Could you check a few things on this model? Use its own coordinates, in mm. A direction names the side the tool comes from. Give positions to 0.01 mm unless a question says otherwise; leave off trailing zeros. Loops run counter-clockwise (first coordinate to the right, second up) from the corner with the lowest first, then second, coordinate; pieces in that order, holes last.
1. Imagine slicing it at D-D (x = -3.25). List the corners of the cut face in (y, z) for me, plus the area to 3 significant figures.
2. Imagine slicing it at A-A (y = 1.5). List the corners of the cut face in (x, z) for me, plus the area to 3 significant figures.
3. Thinking about a two-plate mould opening in X: for faces 1 (the flat face through (0, 0, 0)), 2 (the flat face through (-1.5, -7, 0)), 3 (the flat face through (2, -4, 0)), 4 (the flat face through (1.5, -7, 0)), which applies, +X half, -X half, draft (parallel to the pull), parting line (faces both ways), or undercut?
4. Imagine slicing it at B-B (z = 0). List the corners of the cut face in (x, y) for me, plus the area to 3 significant figures.
5. For faces 5 (the flat face through (-2, -2, -2)), 6 (the flat face through (0, -10, 0)), 7 (the flat face through (-2, -4, 0)), which set-ups out of +Z, -Z, +X, -X, +Y, -Y let a thin tool reach every point of the face, with its end or its side?
6. I need wall thicknesses on line 1 along X through (y, z) = (-7.5, 1.5); line 2 along Y through (x, z) = (2, 1); line 3 along Y through (x, z) = (0, 0). Which ranges of each line are inside material? Lowest first, please.
7. Imagine slicing it at C-C (y = -1). List the corners of the cut face in (x, z) for me, plus the area to 3 significant figures.
8. For P1, Ø1.5, axis at x = 2, z = 3.5, coming from the -Y side; P2, Ø4, axis at y = -7.5, z = -0.5, coming from the +X side; P3, Ø0.5, axis at x = -2, z = 0.5, coming from the -Y side; P4, Ø1.5, axis at x = -3, y = -6, coming from the -Z side, each with a flat end and sliding along its axis, tell me the tip position at first contact or that it passes through.
```python
from build123d import *

# Parameters (mm, degrees)
SKETCH1_R           = 3.95
BOSS_EXTRUDE1_DEPTH = 4
SKETCH2_R           = 4.4
BOSS_EXTRUDE2_DEPTH = 2
SKETCH4_R           = 2.4
BOSS_EXTRUDE3_DEPTH = 2
BOSS_EXTRUDE4_DEPTH = 6
SKETCH6_R           = 4.4
SKETCH6_R_2         = 3.95
BOSS_EXTRUDE5_DEPTH = 4
CUT_EXTRUDE1_DEPTH  = 4


with BuildPart() as part:
    # Sketch1 → Boss-Extrude1 (new body)
    with BuildSketch(Plane(origin=(0, 0, 0), x_dir=(1, 0, 0), z_dir=(0, 1, 0))):
        with Locations(Location((0, 0, 0), (0, 0, 270))):
            Circle(SKETCH1_R)
        with BuildLine():
            ThreePointArc((-0.166646614, 2.345141313), (-0.092401566, 2.286261662), (0, 2.2652595))
            ThreePointArc((0, 2.2652595), (0.092401566, 2.286261662), (0.166646614, 2.345141313))
            ThreePointArc((0.166646614, 2.345141313), (0.365153552, 2.422635524), (0.531999564, 2.290073216))
            ThreePointArc((0.531999564, 2.290073216), (0.585591031, 2.211925311), (0.667696959, 2.164620376))
            ThreePointArc((0.667696959, 2.164620376), (0.762183879, 2.157453631), (0.850485509, 2.191833312))
            ThreePointArc((0.850485509, 2.191833312), (1.063015161, 2.207373726), (1.183375246, 2.031522064))
            ThreePointArc((1.183375246, 2.031522064), (1.211551295, 1.941049689), (1.276066113, 1.871645232))
            ThreePointArc((1.276066113, 1.871645232), (1.364242809, 1.836946378), (1.458755034, 1.843771303))
            ThreePointArc((1.458755034, 1.843771303), (1.666423208, 1.795977086), (1.729602845, 1.592461261))
            ThreePointArc((1.729602845, 1.592461261), (1.72985991, 1.497703284), (1.771051193, 1.412366197))
            ThreePointArc((1.771051193, 1.412366197), (1.845082779, 1.353218377), (1.937407773, 1.331882123))
            ThreePointArc((1.937407773, 1.331882123), (2.121762239, 1.225), (2.12214764, 1.011903287))
            ThreePointArc((2.12214764, 1.011903287), (2.094462881, 0.92127937), (2.108670602, 0.827592226))
            ThreePointArc((2.108670602, 0.827592226), (2.161979047, 0.749250985), (2.243913329, 0.701649371))
            ThreePointArc((2.243913329, 0.701649371), (2.388573385, 0.545176288), (2.326130305, 0.341433266))
            ThreePointArc((2.326130305, 0.341433266), (2.272963633, 0.262995741), (2.258925375, 0.169283054))
            ThreePointArc((2.258925375, 0.169283054), (2.286773988, 0.078709355), (2.351037339, 0.009071994))
            ThreePointArc((2.351037339, 0.009071994), (2.443149303, -0.183088729), (2.323426084, -0.3593746))
            ThreePointArc((2.323426084, -0.3593746), (2.249501592, -0.418656214), (2.208464714, -0.504067659))
            ThreePointArc((2.208464714, -0.504067659), (2.208379026, -0.598825947), (2.249261363, -0.68431147))
            ThreePointArc((2.249261363, -0.68431147), (2.280640684, -0.89508551), (2.114275259, -1.028250455))
            ThreePointArc((2.114275259, -1.028250455), (2.026161462, -1.063108727), (1.961772273, -1.13262975))
            ThreePointArc((1.961772273, -1.13262975), (1.933759896, -1.223152935), (1.947628645, -1.316890857))
            ThreePointArc((1.947628645, -1.316890857), (1.915487132, -1.527550015), (1.717261799, -1.605761745))
            ThreePointArc((1.717261799, -1.605761745), (1.622787995, -1.613099364), (1.540767756, -1.660552716))
            ThreePointArc((1.540767756, -1.660552716), (1.487317713, -1.738797417), (1.472940575, -1.832458712))
            ThreePointArc((1.472940575, -1.832458712), (1.380134142, -2.024284997), (1.167662092, -2.040594058))
            ThreePointArc((1.167662092, -2.040594058), (1.075222693, -2.019759044), (0.982859262, -2.040928287))
            ThreePointArc((0.982859262, -2.040928287), (0.908720824, -2.099942118), (0.86737527, -2.185204569))
            ThreePointArc((0.86737527, -2.185204569), (0.722150177, -2.341153374), (0.514310485, -2.294110633))
            ThreePointArc((0.514310485, -2.294110633), (0.432119136, -2.246954269), (0.337619409, -2.239958423))
            ThreePointArc((0.337619409, -2.239958423), (0.249380102, -2.274497747), (0.184739867, -2.343785411))
            ThreePointArc((0.184739867, -2.343785411), (0, -2.45), (-0.184739867, -2.343785411))
            ThreePointArc((-0.184739867, -2.343785411), (-0.249380102, -2.274497747), (-0.337619409, -2.239958423))
            ThreePointArc((-0.337619409, -2.239958423), (-0.432119136, -2.246954269), (-0.514310485, -2.294110633))
            ThreePointArc((-0.514310485, -2.294110633), (-0.722150177, -2.341153374), (-0.86737527, -2.185204569))
            ThreePointArc((-0.86737527, -2.185204569), (-0.908720824, -2.099942118), (-0.982859262, -2.040928287))
            ThreePointArc((-0.982859262, -2.040928287), (-1.075222693, -2.019759044), (-1.167662092, -2.040594058))
            ThreePointArc((-1.167662092, -2.040594058), (-1.380134142, -2.024284997), (-1.472940575, -1.832458712))
            ThreePointArc((-1.472940575, -1.832458712), (-1.487317713, -1.738797417), (-1.540767756, -1.660552716))
            ThreePointArc((-1.540767756, -1.660552716), (-1.622787995, -1.613099364), (-1.717261799, -1.605761745))
            ThreePointArc((-1.717261799, -1.605761745), (-1.915487132, -1.527550015), (-1.947628645, -1.316890857))
            ThreePointArc((-1.947628645, -1.316890857), (-1.933759896, -1.223152935), (-1.961772273, -1.13262975))
            ThreePointArc((-1.961772273, -1.13262975), (-2.026161462, -1.063108727), (-2.114275259, -1.028250455))
            ThreePointArc((-2.114275259, -1.028250455), (-2.280640684, -0.89508551), (-2.249261363, -0.68431147))
            ThreePointArc((-2.249261363, -0.68431147), (-2.208379026, -0.598825947), (-2.208464714, -0.504067659))
            ThreePointArc((-2.208464714, -0.504067659), (-2.249501592, -0.418656214), (-2.323426084, -0.3593746))
            ThreePointArc((-2.323426084, -0.3593746), (-2.443149303, -0.183088729), (-2.351037339, 0.009071994))
            ThreePointArc((-2.351037339, 0.009071994), (-2.286773988, 0.078709355), (-2.258925375, 0.169283054))
            ThreePointArc((-2.258925375, 0.169283054), (-2.272963633, 0.262995741), (-2.326130305, 0.341433266))
            ThreePointArc((-2.326130305, 0.341433266), (-2.388573385, 0.545176288), (-2.243913329, 0.701649371))
            ThreePointArc((-2.243913329, 0.701649371), (-2.161979047, 0.749250985), (-2.108670602, 0.827592226))
            ThreePointArc((-2.108670602, 0.827592226), (-2.094462881, 0.92127937), (-2.12214764, 1.011903287))
            ThreePointArc((-2.12214764, 1.011903287), (-2.121762239, 1.225), (-1.937407773, 1.331882123))
            ThreePointArc((-1.937407773, 1.331882123), (-1.845082779, 1.353218377), (-1.771051193, 1.412366197))
            ThreePointArc((-1.771051193, 1.412366197), (-1.72985991, 1.497703284), (-1.729602845, 1.592461261))
            ThreePointArc((-1.729602845, 1.592461261), (-1.666423208, 1.795977086), (-1.458755034, 1.843771303))
            ThreePointArc((-1.458755034, 1.843771303), (-1.364242809, 1.836946378), (-1.276066113, 1.871645232))
            ThreePointArc((-1.276066113, 1.871645232), (-1.211551295, 1.941049689), (-1.183375246, 2.031522064))
            ThreePointArc((-1.183375246, 2.031522064), (-1.063015161, 2.207373726), (-0.850485509, 2.191833312))
            ThreePointArc((-0.850485509, 2.191833312), (-0.762183879, 2.157453631), (-0.667696959, 2.164620376))
            ThreePointArc((-0.667696959, 2.164620376), (-0.585591031, 2.211925311), (-0.531999564, 2.290073216))
            ThreePointArc((-0.531999564, 2.290073216), (-0.365153552, 2.422635524), (-0.166646614, 2.345141313))
        make_face(mode=Mode.SUBTRACT)
    extrude(amount=BOSS_EXTRUDE1_DEPTH)

    # Sketch2 → Boss-Extrude2 (add)
    with BuildSketch(Plane.XZ):
        with Locations(Location((0, 0, 0), (0, 0, 270))):
            Circle(SKETCH2_R)
    extrude(amount=BOSS_EXTRUDE2_DEPTH)

    # Sketch4 → Boss-Extrude3 (add)
    with BuildSketch(Plane.XZ.offset(2)):
        with Locations(Location((0, 0, 0), (0, 0, 270))):
            Circle(SKETCH4_R)
    extrude(amount=BOSS_EXTRUDE3_DEPTH)

    # Sketch5 → Boss-Extrude4 (add)
    with BuildSketch(Plane.XZ.offset(4)):
        with BuildLine():
            ThreePointArc((1.5, 1.8734994), (0, 2.4), (-1.5, 1.8734994))
            Line((-1.5, 1.8734994), (-1.5, -1.8734994))
            ThreePointArc((-1.5, -1.8734994), (0, -2.4), (1.5, -1.8734994))
            Line((1.5, -1.8734994), (1.5, 1.8734994))
        make_face()
    extrude(amount=BOSS_EXTRUDE4_DEPTH)

    # Sketch6 → Boss-Extrude5 (add)
    with BuildSketch(Plane(origin=(0, 0, 0), x_dir=(1, 0, 0), z_dir=(0, 1, 0))):
        with Locations(Location((0, 0, 0), (0, 0, 270))):
            Circle(SKETCH6_R)
        Circle(SKETCH6_R_2, mode=Mode.SUBTRACT)
    extrude(amount=BOSS_EXTRUDE5_DEPTH)

    # Sketch8 → Cut-Extrude1 (cut)
    with BuildSketch(Plane(origin=(0, 4, 0), x_dir=(1, 0, 0), z_dir=(0, 1, 0))):
        with BuildLine():
            ThreePointArc((0.746832801, 2.421172474), (0.402414119, 2.669843231), (0, 2.533739407))
            ThreePointArc((0, 2.533739407), (-0.402414119, 2.669843231), (-0.746832801, 2.421172474))
            ThreePointArc((-0.746832801, 2.421172474), (-1.171486096, 2.432615943), (-1.42730623, 2.093473742))
            ThreePointArc((-1.42730623, 2.093473742), (-1.836466392, 1.979240054), (-1.980957237, 1.579760681))
            ThreePointArc((-1.980957237, 1.579760681), (-2.33826859, 1.35), (-2.3585915, 0.92567895))
            ThreePointArc((-2.3585915, 0.92567895), (-2.632305363, 0.600806522), (-2.526654558, 0.189346583))
            ThreePointArc((-2.526654558, 0.189346583), (-2.692450252, -0.201771253), (-2.47021327, -0.563810059))
            ThreePointArc((-2.47021327, -0.563810059), (-2.513359121, -0.986420766), (-2.194282693, -1.266869704))
            ThreePointArc((-2.194282693, -1.266869704), (-2.110945003, -1.683422465), (-1.723380469, -1.857362415))
            ThreePointArc((-1.723380469, -1.857362415), (-1.520964157, -2.230844691), (-1.099348328, -2.282820325))
            ThreePointArc((-1.099348328, -2.282820325), (-0.795838971, -2.580046576), (-0.377634263, -2.505439631))
            ThreePointArc((-0.377634263, -2.505439631), (0, -2.7), (0.377634263, -2.505439631))
            ThreePointArc((0.377634263, -2.505439631), (0.795838971, -2.580046576), (1.099348328, -2.282820325))
            ThreePointArc((1.099348328, -2.282820325), (1.520964157, -2.230844691), (1.723380469, -1.857362415))
            ThreePointArc((1.723380469, -1.857362415), (2.110945003, -1.683422465), (2.194282693, -1.266869704))
            ThreePointArc((2.194282693, -1.266869704), (2.513359121, -0.986420766), (2.47021327, -0.563810059))
            ThreePointArc((2.47021327, -0.563810059), (2.692450252, -0.201771253), (2.526654558, 0.189346583))
            ThreePointArc((2.526654558, 0.189346583), (2.632305363, 0.600806522), (2.3585915, 0.92567895))
            ThreePointArc((2.3585915, 0.92567895), (2.33826859, 1.35), (1.980957237, 1.579760681))
            ThreePointArc((1.980957237, 1.579760681), (1.836466392, 1.979240054), (1.42730623, 2.093473742))
            ThreePointArc((1.42730623, 2.093473742), (1.171486096, 2.432615943), (0.746832801, 2.421172474))
        make_face()
    extrude(amount=-CUT_EXTRUDE1_DEPTH, mode=Mode.SUBTRACT)


solid = part.part
```
Derived:
1. outline: (-2, -2.97) - (4, -2.97) - (4, 2.97) - (-2, 2.97) - close
1. area: 35.6 mm2
2. outline: circle Ø8.8 at (0, 0); hole (-2.53, -0.19) arc R0.46 ccw to (-2.36, -0.93) arc R0.46 ccw to (-1.98, -1.58) arc R0.46 ccw to (-1.43, -2.09) arc R0.46 ccw to (-0.75, -2.42) arc R0.46 ccw to (0, -2.53) arc R0.46 ccw to (0.75, -2.42) arc R0.46 ccw to (1.43, -2.09) arc R0.46 ccw to (1.98, -1.58) arc R0.46 ccw to (2.36, -0.93) arc R0.46 ccw to (2.53, -0.19) arc R0.46 ccw to (2.47, 0.56) arc R0.46 ccw to (2.19, 1.27) arc R0.46 ccw to (1.72, 1.86) arc R0.46 ccw to (1.1, 2.28) arc R0.46 ccw to (0.38, 2.51) arc R0.46 ccw to (-0.38, 2.51) arc R0.46 ccw to (-1.1, 2.28) arc R0.46 ccw to (-1.72, 1.86) arc R0.46 ccw to (-2.19, 1.27) arc R0.46 ccw to (-2.47, 0.56) arc R0.46 ccw to start
2. area: 38.8 mm2
3. face 1: undercut
3. face 2: -X half
3. face 3: draft
3. face 4: +X half
4. outline: (-4.4, -2) - (-2.4, -2) - (-2.4, -4) - (-1.5, -4) - (-1.5, -10) - (1.5, -10) - (1.5, -4) - (2.4, -4) - (2.4, -2) - (4.4, -2) - (4.4, 4) - (2.66, 4) - (2.66, 0) - (-2.66, 0) - (-2.66, 4) - (-4.4, 4) - close
4. area: 59.1 mm2
5. face 5: -Y
5. face 6: +Z, -Z, +X, -X, -Y
5. face 7: +Z, -Z, -X, -Y
6. line 1: x = -1.5 to 1.5
6. line 2: y = -4 to 0
6. line 3: y = -10 to 0
7. outline: circle Ø8.8 at (0, 0)
7. area: 60.8 mm2
8. P1: stops at y = -2
8. P2: stops at x = 1.5
8. P3: stops at y = -4
8. P4: passes through
